```python
from build123d import *

# Parameters (mm, degrees)
BASE_FLANGE1_DEPTH = 199
CUT_EXTRUDE1_REACH = 224.823
SKETCH6_R          = 4.15
FILLET1_R          = 3
CUT_EXTRUDE2_REACH = 225.273
SKETCH8_R          = 45.15
SKETCH8_R_2        = 4.15


# Sheet-metal steps are written as plain solids
with BuildPart() as part:
    # Sketch1 → Base-Flange1 (new, symmetric)
    with BuildSketch(Plane.XY):
        with BuildLine():
            Line((-95, 0), (-69.5, 0))
            ThreePointArc((-69.5, 0), (-66.318019485, 1.318019485), (-65, 4.5))
            Line((-65, 4.5), (-65, 30.5))
            ThreePointArc((-65, 30.5), (-64.560660172, 31.560660172), (-63.5, 32))
            Line((-63.5, 32), (63.5, 32))
            ThreePointArc((63.5, 32), (64.560660172, 31.560660172), (65, 30.5))
            Line((65, 30.5), (65, 4.5))
            ThreePointArc((65, 4.5), (66.318019485, 1.318019485), (69.5, 0))
            Line((69.5, 0), (95, 0))
            Line((95, 0), (95, 3))
            Line((95, 3), (69.5, 3))
            ThreePointArc((69.5, 3), (68.439339828, 3.439339828), (68, 4.5))
            Line((68, 4.5), (68, 30.5))
            ThreePointArc((68, 30.5), (66.681980515, 33.681980515), (63.5, 35))
            Line((63.5, 35), (-63.5, 35))
            ThreePointArc((-63.5, 35), (-66.681980515, 33.681980515), (-68, 30.5))
            Line((-68, 30.5), (-68, 4.5))
            ThreePointArc((-68, 4.5), (-68.439339828, 3.439339828), (-69.5, 3))
            Line((-69.5, 3), (-95, 3))
            Line((-95, 3), (-95, 0))
        make_face()
    extrude(amount=BASE_FLANGE1_DEPTH, both=True)

    # Sketch6 → Cut-Extrude1 (cut, up to next)
    with BuildSketch(Plane(origin=(0, 3, 0), x_dir=(1, 0, 0), z_dir=(0, 1, 0)), mode=Mode.PRIVATE) as cut_extrude1_sk1:
        with Locations(Location((-83, -184, 0), (0, 0, 180))):
            Circle(SKETCH6_R)
    cut_extrude1_tool1 = extrude(cut_extrude1_sk1.sketch, amount=-CUT_EXTRUDE1_REACH, mode=Mode.PRIVATE) & part.part
    # Sketch6 → Cut-Extrude1 (cut, up to next)
    with BuildSketch(Plane(origin=(0, 3, 0), x_dir=(1, 0, 0), z_dir=(0, 1, 0)), mode=Mode.PRIVATE) as cut_extrude1_sk2:
        with Locations(Location((-83, 54, 0), (0, 0, 180))):
            Circle(SKETCH6_R)
    cut_extrude1_tool2 = extrude(cut_extrude1_sk2.sketch, amount=-CUT_EXTRUDE1_REACH, mode=Mode.PRIVATE) & part.part
    # Sketch6 → Cut-Extrude1 (cut, up to next)
    with BuildSketch(Plane(origin=(0, 3, 0), x_dir=(1, 0, 0), z_dir=(0, 1, 0)), mode=Mode.PRIVATE) as cut_extrude1_sk3:
        with Locations(Location((-83, 184, 0), (0, 0, 180))):
            Circle(SKETCH6_R)
    cut_extrude1_tool3 = extrude(cut_extrude1_sk3.sketch, amount=-CUT_EXTRUDE1_REACH, mode=Mode.PRIVATE) & part.part
    # Sketch6 → Cut-Extrude1 (cut, up to next)
    with BuildSketch(Plane(origin=(0, 3, 0), x_dir=(1, 0, 0), z_dir=(0, 1, 0)), mode=Mode.PRIVATE) as cut_extrude1_sk4:
        with Locations((83, 184)):
            Circle(SKETCH6_R)
    cut_extrude1_tool4 = extrude(cut_extrude1_sk4.sketch, amount=-CUT_EXTRUDE1_REACH, mode=Mode.PRIVATE) & part.part
    # Sketch6 → Cut-Extrude1 (cut, up to next)
    with BuildSketch(Plane(origin=(0, 3, 0), x_dir=(1, 0, 0), z_dir=(0, 1, 0)), mode=Mode.PRIVATE) as cut_extrude1_sk5:
        with Locations((83, 54)):
            Circle(SKETCH6_R)
    cut_extrude1_tool5 = extrude(cut_extrude1_sk5.sketch, amount=-CUT_EXTRUDE1_REACH, mode=Mode.PRIVATE) & part.part
    # Sketch6 → Cut-Extrude1 (cut, up to next)
    with BuildSketch(Plane(origin=(0, 3, 0), x_dir=(1, 0, 0), z_dir=(0, 1, 0)), mode=Mode.PRIVATE) as cut_extrude1_sk6:
        with Locations((83, -184)):
            Circle(SKETCH6_R)
    cut_extrude1_tool6 = extrude(cut_extrude1_sk6.sketch, amount=-CUT_EXTRUDE1_REACH, mode=Mode.PRIVATE) & part.part
    add(cut_extrude1_tool1.solids().sort_by_distance((-83, 3, 184))[0], mode=Mode.SUBTRACT)
    add(cut_extrude1_tool2.solids().sort_by_distance((-83, 3, -54))[0], mode=Mode.SUBTRACT)
    add(cut_extrude1_tool3.solids().sort_by_distance((-83, 3, -184))[0], mode=Mode.SUBTRACT)
    add(cut_extrude1_tool4.solids().sort_by_distance((83, 3, -184))[0], mode=Mode.SUBTRACT)
    add(cut_extrude1_tool5.solids().sort_by_distance((83, 3, -54))[0], mode=Mode.SUBTRACT)
    add(cut_extrude1_tool6.solids().sort_by_distance((83, 3, 184))[0], mode=Mode.SUBTRACT)

    # Fillet1
    fillet1_edges = [part.edges().sort_by_distance(p)[0] for p in [
        (95, 1.5, -199),
        (-95, 1.5, -199),
        (95, 1.5, 199),
        (-95, 1.5, 199),
    ]]
    fillet(fillet1_edges, radius=FILLET1_R)

    # Sketch8 → Cut-Extrude2 (cut, up to next)
    with BuildSketch(Plane(origin=(0, 35, 0), x_dir=(1, 0, 0), z_dir=(0, 1, 0)), mode=Mode.PRIVATE) as cut_extrude2_sk1:
        with Locations(Location((0, -126, 0), (0, 0, 270))):
            Circle(SKETCH8_R)
    cut_extrude2_tool1 = extrude(cut_extrude2_sk1.sketch, amount=-CUT_EXTRUDE2_REACH, mode=Mode.PRIVATE) & part.part
    # Sketch8 → Cut-Extrude2 (cut, up to next)
    with BuildSketch(Plane(origin=(0, 35, 0), x_dir=(1, 0, 0), z_dir=(0, 1, 0)), mode=Mode.PRIVATE) as cut_extrude2_sk2:
        with Locations(Location((-42.426406871, -83.573593129, 0), (0, 0, 270))):
            Circle(SKETCH8_R_2)
    cut_extrude2_tool2 = extrude(cut_extrude2_sk2.sketch, amount=-CUT_EXTRUDE2_REACH, mode=Mode.PRIVATE) & part.part
    # Sketch8 → Cut-Extrude2 (cut, up to next)
    with BuildSketch(Plane(origin=(0, 35, 0), x_dir=(1, 0, 0), z_dir=(0, 1, 0)), mode=Mode.PRIVATE) as cut_extrude2_sk3:
        with Locations(Location((42.426406871, -83.573593129, 0), (0, 0, 270))):
            Circle(SKETCH8_R_2)
    cut_extrude2_tool3 = extrude(cut_extrude2_sk3.sketch, amount=-CUT_EXTRUDE2_REACH, mode=Mode.PRIVATE) & part.part
    # Sketch8 → Cut-Extrude2 (cut, up to next)
    with BuildSketch(Plane(origin=(0, 35, 0), x_dir=(1, 0, 0), z_dir=(0, 1, 0)), mode=Mode.PRIVATE) as cut_extrude2_sk4:
        with Locations(Location((42.426406871, -168.426406871, 0), (0, 0, 270))):
            Circle(SKETCH8_R_2)
    cut_extrude2_tool4 = extrude(cut_extrude2_sk4.sketch, amount=-CUT_EXTRUDE2_REACH, mode=Mode.PRIVATE) & part.part
    # Sketch8 → Cut-Extrude2 (cut, up to next)
    with BuildSketch(Plane(origin=(0, 35, 0), x_dir=(1, 0, 0), z_dir=(0, 1, 0)), mode=Mode.PRIVATE) as cut_extrude2_sk5:
        with Locations(Location((-42.426406871, -168.426406871, 0), (0, 0, 270))):
            Circle(SKETCH8_R_2)
    cut_extrude2_tool5 = extrude(cut_extrude2_sk5.sketch, amount=-CUT_EXTRUDE2_REACH, mode=Mode.PRIVATE) & part.part
    add(cut_extrude2_tool1.solids().sort_by_distance((0, 35, 126))[0], mode=Mode.SUBTRACT)
    add(cut_extrude2_tool2.solids().sort_by_distance((-42.426407, 35, 83.573593))[0], mode=Mode.SUBTRACT)
    add(cut_extrude2_tool3.solids().sort_by_distance((42.426407, 35, 83.573593))[0], mode=Mode.SUBTRACT)
    add(cut_extrude2_tool4.solids().sort_by_distance((42.426407, 35, 168.426407))[0], mode=Mode.SUBTRACT)
    add(cut_extrude2_tool5.solids().sort_by_distance((-42.426407, 35, 168.426407))[0], mode=Mode.SUBTRACT)


solid = part.part
```
Work out the finished part from the listing and answer in its coordinate system (mm). A direction names the side the tool comes from. Coordinates: 2 decimals unless noted, no trailing zeros. Write each loop counter-clockwise with the first axis right and the second up, starting at its lowest first coordinate (ties: lowest second). Pieces come first, ordered by that corner, then holes. Notation, with made-up numbers: (11, -21.75) - (57, -21.75) arc R17 ccw to (57, -6.75) - close; hole circle Ø8 at (-30, 82.25). An arc over 180 degrees is marked (long way). Answer as a JSON object with one key per item and string values.
Q1. Find section A-A (z = 184). Write down the section's boundary in (x, y), plus the area to 3 significant figures.
Results list:
{"outline": "(-95, 0) - (-87.15, 0) - (-87.15, 3) - (-95, 3) - close; (-78.85, 0) - (-69.5, 0) arc R4.5 ccw to (-65, 4.5) - (-65, 30.5) arc R1.5 cw to (-63.5, 32) - (63.5, 32) arc R1.5 cw to (65, 30.5) - (65, 4.5) arc R4.5 ccw to (69.5, 0) - (78.85, 0) - (78.85, 3) - (69.5, 3) arc R1.5 cw to (68, 4.5) - (68, 30.5) arc R4.5 ccw to (63.5, 35) - (-63.5, 35) arc R4.5 ccw to (-68, 30.5) - (-68, 4.5) arc R1.5 cw to (-69.5, 3) - (-78.85, 3) - close; (87.15, 0) - (95, 0) - (95, 3) - (87.15, 3) - close", "area": "697 mm^2"}
Q2. Find section D-D (y = 12). Write down the section's boundary in (x, z).
Results list:
{"outline": "(-68, -199) - (-65, -199) - (-65, 199) - (-68, 199) - close; (65, -199) - (68, -199) - (68, 199) - (65, 199) - close"}
Q3. Given pin 1 Ø5 at (x, z) = (-40.5, 117.5) entering from -Y; pin 2 Ø4 at (y, z) = (18.5, -115.5) entering from +X; pin 3 Ø8 at (y, z) = (28, -90.5) entering from -X; pin 4 Ø20.5 at (x, z) = (-79, -56.5) entering from +Y, each flat-ended and moving along its own axis, determine where each tip first touches the part or whether it passes through.
Results list:
{"pin 1": "passes through", "pin 2": "stops at x = 68", "pin 3": "stops at x = -68", "pin 4": "stops at y = 3.2"}
Q4. Consider L1, parallel to Z at x = 83, y = 0.7; L2, parallel to X at y = 25, z = -46; L3, parallel to Y at x = -20, z = -15. Determine where each line is inside the solid, lowest interval first. Write a range as from..to.
Results list:
{"L1": "z = -199..-188.15, -179.85..-58.15, -49.85..179.85, 188.15..199", "L2": "x = -68..-65, 65..68", "L3": "y = 32..35"}
Q5. Find section B-B (x = 24). Write down the section's boundary in (y, z), plus the area to 3 significant figures.
Results list:
{"outline": "(32, -199) - (35, -199) - (35, 87.76) - (32, 87.76) - close; (32, 164.24) - (35, 164.24) - (35, 199) - (32, 199) - close", "area": "965 mm^2"}
Q6. For a pull along X with two mould halves and no side action, classify faces 1 (the flat face through (-65, 17, 3)), 2 (the flat face through (65, 18, 3)), 3 (the flat face through (-82, 3, 3)), 4 (the flat face through (-68, 18, 3)) as pulls with the +X half, pulls with the -X half, needs draft (parallel to the pull), parting line crosses it, or undercut.
Results list:
{"face 1": "undercut", "face 2": "undercut", "face 3": "needs draft", "face 4": "pulls with the -X half"}
Q7. Which of the six approach directions +Z, -Z, +X, -X, +Y, -Y give full straight-line access (tool end or side, diameter ignored) to faces 5 (the cylindrical face through (82.1, 1.52, 188.05)), 6 (the flat face through (-1, 32, 3)), 7 (the flat face through (82, 3, 3))?
Results list:
{"face 5": "+Y, -Y", "face 6": "+Z, -Z, -Y", "face 7": "+Z, -Z, +X, +Y"}
Q8. Find section C-C (z = 126). Write down the section's boundary in (x, y), plus the area to 3 significant figures.
Results list:
{"outline": "(-95, 0) - (-69.5, 0) arc R4.5 ccw to (-65, 4.5) - (-65, 30.5) arc R1.5 cw to (-63.5, 32) - (-45.15, 32) - (-45.15, 35) - (-63.5, 35) arc R4.5 ccw to (-68, 30.5) - (-68, 4.5) arc R1.5 cw to (-69.5, 3) - (-95, 3) - close; (45.15, 32) - (63.5, 32) arc R1.5 cw to (65, 30.5) - (65, 4.5) arc R4.5 ccw to (69.5, 0) - (95, 0) - (95, 3) - (69.5, 3) arc R1.5 cw to (68, 4.5) - (68, 30.5) arc R4.5 ccw to (63.5, 35) - (45.15, 35) - close", "area": "476 mm^2"}
